Check sheet for the modelled part. Datum: model origin and axes. Units: mm. Face numbers are marked on the shaded views. A direction names the side the tool comes from. Round coordinates to 2 decimals unless told otherwise and drop trailing zeros. Order: outer loops, then holes, each group sorted by start corner. A loop starts at its lowest first (then second) coordinate and runs counter-clockwise, first axis right, second up.
```python
from build123d import *

# Parameters (mm, degrees)
F1_DEPTH = 10
F2_W     = 4.5
F2_H     = 4.5
F3_DEPTH = 4.5
F4_W     = 4.5
F4_H     = 4.5
F5_DEPTH = 4.5


with BuildPart() as f1:
    # F0 (on Front) → F1 (new body)
    with BuildSketch(Plane.XZ):
        Polygon((25.658527257, 23.514753694), (-25.441472743, 23.514753694), (-18.9181555508, -17.6718501088), (-40.9436055461, -14.1833615384), (-40.9436055461, -46.6833615384), (-28.9440269134, -46.7839231504), (0, 15.8518757671), (29.1606600601, -46.6833615384), (41.1606600601, -46.6833615384), (41.1606600601, -14.1833615384), (19.1352100648, -17.6718501088), align=None)
    extrude(amount=F1_DEPTH)

    # F2 (on face) → F3 (join)
    with BuildSketch(Plane(origin=(-0.3940744361, 0, -47.0231839888), x_dir=(0.9999648861, 0, -0.0083801343), z_dir=(-0.0083801343, 0, -0.9999648861))):
        with Locations((-36.2935631948, 5.5205655236)):
            Rectangle(F2_W, F2_H)
    extrude(amount=F3_DEPTH)

    # F4 (on face) → F5 (join)
    with BuildSketch(Plane(origin=(0, 0, -46.6833615384), x_dir=(1, 0, 0), z_dir=(0, 0, -1))):
        with Locations((36.903268241, 5.5205655236)):
            Rectangle(F4_W, F4_H)
    extrude(amount=F5_DEPTH)


solid = f1.part
```
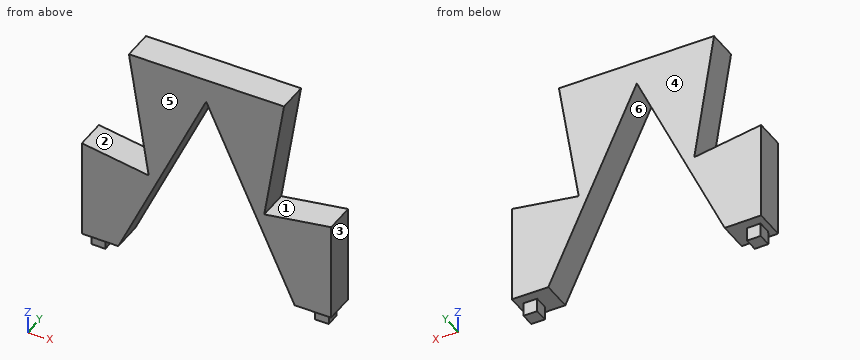
Item 1: Sectioned sample at D-D (y = -1.75). Record the cut outline in (x, z), and give its area (3 significant figures).
Answer:
outline: (-40.94, -46.68) - (-28.94, -46.78) - (0, 15.85) - (29.16, -46.68) - (41.16, -46.68) - (41.16, -14.18) - (19.14, -17.67) - (25.66, 23.51) - (-25.44, 23.51) - (-18.92, -17.67) - (-40.94, -14.18) - close
area: 2,480 mm2
Item 2: Access from +Z, -Z, +X, -X, +Y, -Y to the whole of each face (thin tool, end or side, straight path). Record for the marked faces 5 and 6.
Answer:
face 5: +Z, -Z, +X, -X, -Y
face 6: -Z, +Y, -Y
Item 3: Release check for a two-part mould opening along X. For the marked faces 1, 2, 3 and 4 record: released by +X, released by -X, zero draft, split by the parting line, or undercut.
Answer:
face 1: undercut
face 2: undercut
face 3: released by +X
face 4: zero draft
Item 4: Scan lines: line 1 along X through (y, z) = (-4, -34); line 2 along Z through (x, y) = (14, -5.5); line 3 along X through (y, z) = (-8.5, 15). Record each from-to range of solid material in increasing order.
Answer:
line 1: x = -40.94 to -23.04, 23.25 to 41.16
line 2: z = -14.17 to 23.51
line 3: x = -24.09 to -0.39, 0.4 to 24.31
Item 5: Sectioned sample at C-C (x = -22). Record the cut outline in (y, z).
Answer:
outline: (-10, -31.76) - (0, -31.76) - (0, -17.18) - (-10, -17.18) - close; (-10, 1.79) - (0, 1.79) - (0, 23.51) - (-10, 23.51) - close
Item 6: Go/stop test with flat-tipped pins: P1, Ø1.3, axis at x = 37.5, z = -48.5, coming from the +Y side; P2, Ø3, axis at x = 17.5, y = -1.5, coming from the -Z side; P3, Ø3.5, axis at y = -5.5, z = -48.5, coming from the +X side. Record where each tip stops, or that it passes through.
Answer:
P1: stops at y = -3.27
P2: stops at z = -24.89
P3: stops at x = 39.15
Item 7: Sectioned sample at B-B (z = -21.5). Record the cut outline in (x, y), and give its area (3 significant figures).
Answer:
outline: (-40.94, -10) - (-17.26, -10) - (-17.26, 0) - (-40.94, 0) - close; (17.42, -10) - (41.16, -10) - (41.16, 0) - (17.42, 0) - close
area: 474 mm2
Item 8: Sectioned sample at A-A (y = -6). Record the cut outline in (x, z), and give its area (3 significant figures).
Answer:
outline: (-40.94, -46.68) - (-38.94, -46.7) - (-38.97, -51.2) - (-34.47, -51.24) - (-34.44, -46.74) - (-28.94, -46.78) - (0, 15.85) - (29.16, -46.68) - (34.65, -46.68) - (34.65, -51.18) - (39.15, -51.18) - (39.15, -46.68) - (41.16, -46.68) - (41.16, -14.18) - (19.14, -17.67) - (25.66, 23.51) - (-25.44, 23.51) - (-18.92, -17.67) - (-40.94, -14.18) - close
area: 2,520 mm2
